Could you check a few things on this drawing? It's one solid part, dimensions in mm from its lowest x, y, z. Give positions to 0.01 mm unless a question says otherwise; leave off trailing zeros. Loops run counter-clockwise (first coordinate to the right, second up) from the corner with the lowest first, then second, coordinate; pieces in that order, holes last. Notation, with made-up numbers: (-27.5, 36) - (18.5, 36) arc R27 cw to (18.5, 54) - close; hole circle Ø11 at (75, 32.25). An arc over 180 degrees is marked (long way). Use a Markdown table: item, result.
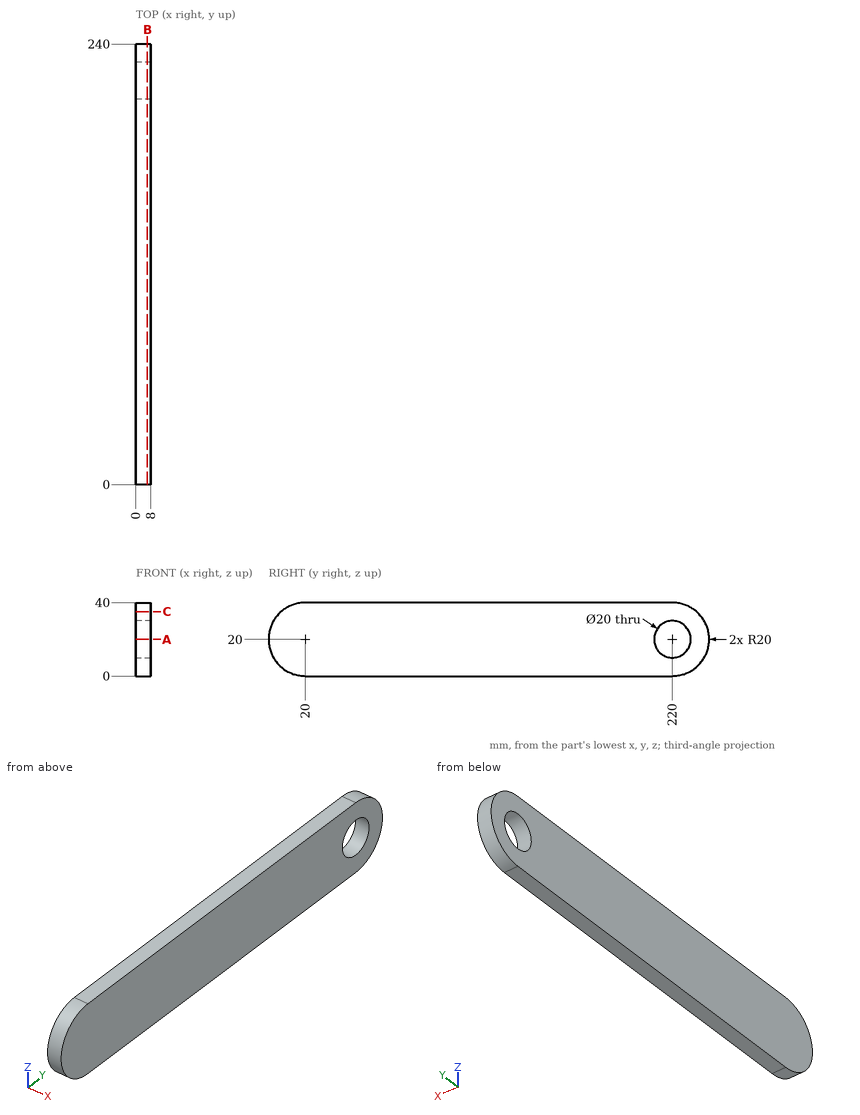
(1) Will these pins go through, and if not, where does the flat tip stop? pin 1 (1 mm diameter, centred on x = 4, z = 5, fed in from -Y) (3 decimals); pin 2 (1.5 mm diameter, centred on x = 5.5, z = 32, fed in from +Y); pin 3 (4 mm diameter, centred on x = 3.5, z = 14, fed in from -Y).
A:
| item | result |
|---|---|
| pin 1 | y = 6.225 |
| pin 2 | y = 236.54 |
| pin 3 | y = 0.4 |
(2) If I drill on line 1 (Y direction, x = 6.25, z = 20); line 2 (Y direction, x = 5.75, z = 27.5); line 3 (Y direction, x = 6.5, z = 6), over which ranges is the centre line in solid material (lowest first)?
A:
| item | result |
|---|---|
| line 1 | 0 to 210, 230 to 240 |
| line 2 | 1.46 to 213.39, 226.61 to 238.54 |
| line 3 | 5.72 to 234.28 |
(3) Suppose I cut it at C-C on z = 35. Write out the boundary of the cut face in (x, y), plus the area to 3 significant figures.
A:
| item | result |
|---|---|
| outline | (0, 6.77) - (8, 6.77) - (8, 233.23) - (0, 233.23) - close |
| area | 1,810 mm2 |
(4) Suppose I cut it at A-A on z = 20. Write out the boundary of the cut face in (x, y).
A:
| item | result |
|---|---|
| outline | (0, 0) - (8, 0) - (8, 210) - (0, 210) - close; (0, 230) - (8, 230) - (8, 240) - (0, 240) - close |
(5) Suppose I cut it at B-B on x = 6.25. Write out the boundary of the cut face in (y, z).
A:
| item | result |
|---|---|
| outline | (20, 0) - (220, 0) arc R20 ccw to (220, 40) - (20, 40) arc R20 ccw to start; hole circle Ø20 at (220, 20) |
